Geometry: final body of the model. Coordinates: model frame, mm. A direction names the side the tool comes from. Round coordinates to 2 decimals unless told otherwise and drop trailing zeros. Write each loop counter-clockwise with the first axis right and the second up, starting at its lowest first coordinate (ties: lowest second). Pieces come first, ordered by that corner, then holes. Notation, with made-up numbers: M 56,22.25 L 69,22.25 A26 ccw 69,61.25 Z; hole C -19,61 d8. An arc over 180 degrees is marked long. Use one line per item in the form item = value. Start each with the question number.
from build123d import *

# Parameters (mm, degrees)
SKETCH_1_R          = 2
EXTRUDE_1_DEPTH     = 24
SKETCH_2_R          = 3
EXTRUDE_2_DEPTH     = 2.5
CUT_EXTRUDE_1_DEPTH = 1.5
FILLET_1_R          = 0.5
CHAMFER_1_SIZE      = 0.5


with BuildPart() as part:
    # 草图1 → 凸台-拉伸1 (new body)
    with BuildSketch(Plane.XY):
        Circle(SKETCH_1_R)
    extrude(amount=EXTRUDE_1_DEPTH)

    # 草图2 → 凸台-拉伸2 (add)
    with BuildSketch(Plane.XY.offset(24)):
        Circle(SKETCH_2_R)
    extrude(amount=EXTRUDE_2_DEPTH)

    # 草图3 → 切除-拉伸1 (cut)
    with BuildSketch(Plane.XY.offset(26.5)):
        Polygon((0, 2.272766295), (-1.968273348, 1.136383147), (-1.968273348, -1.136383147), (0, -2.272766295), (1.968273348, -1.136383147), (1.968273348, 1.136383147), align=None)
    extrude(amount=-CUT_EXTRUDE_1_DEPTH, mode=Mode.SUBTRACT)

    # 圆角1
    fillet_1_edges = [part.edges().sort_by_distance(p)[0] for p in [
        (-3, 0, 26.5),
    ]]
    fillet(fillet_1_edges, radius=FILLET_1_R)

    # 倒角1
    chamfer_1_edges = [part.edges().sort_by_distance(p)[0] for p in [
        (-2, 0, 0),
    ]]
    chamfer(chamfer_1_edges, length=CHAMFER_1_SIZE)


solid = part.part
1. Ray query, probe 1 along Z at (x, y) = (-2.15, -0.05); probe 2 along Z at (x, y) = (-0.95, -0.55); probe 3 along X at (y, z) = (-1.65, 10). Return the intervals inside material, ascending.
2. Pull-direction query (Y, two-part tool) for faces 4 (the face through (0.97, -1.713, 25.76)), 5 (the face through (0, -2, 12)), 6 (the face through (0, 0, 0)); classes: released by +Y, released by -Y, zero draft, split by the parting line, or undercut.
3. Set-up query: faces 1 (the face through (1, -2, 24)), 2 (the face through (-0.998, -1.697, 25.76)), 3 (the face through (-3, 0, 25)). Return all of +Z, -Z, +X, -X, +Y, -Y with unobstructed straight access to the full face (end or side cutting, diameter ignored); none if empty.
4. Section query A-A (y = 0). Return loops of the section in (x, z), then the cut area to 3 significant figures.
5. Section query B-B (z = 6.5). Return loops of the section in (x, y), then the cut area to 3 significant figures.
6. Contact query for flat-ended pins moving along their axis: pin 1 (1 mm diameter, centred on y = 1, z = 5, fed in from -X); pin 2 (3 mm diameter, centred on x = 0, y = 0.5, fed in from +Z); pin 3 (2 mm diameter, centred on x = -0.5, y = 1.5, fed in from +Z); pin 4 (1.5 mm diameter, centred on x = 2, z = 4.5, fed in from +Y). Output: stop coordinate, or through.
Checks:
q1.probe_1 = 24 to 26.5
q1.probe_2 = 0 to 25
q1.probe_3 = -1.13 to 1.13
q2.face_4 = undercut
q2.face_5 = split by the parting line
q2.face_6 = zero draft
q3.face_1 = -Z
q3.face_2 = +Z
q3.face_3 = +Z, -Z
q4.outline = M -3,24 L -2,24 L -2,0.5 L -1.5,0 L 1.5,0 L 2,0.5 L 2,24 L 3,24 L 3,26 A0.5 ccw 2.5,26.5 L 1.97,26.5 L 1.97,25 L -1.97,25 L -1.97,26.5 L -2.5,26.5 A0.5 ccw -3,26 Z
q4.area = 105 mm^2
q5.outline = C 0,0 d4
q5.area = 12.6 mm^2
q6.pin_1 = -1.94
q6.pin_2 = 25
q6.pin_3 = 26.5
q6.pin_4 = 1.56
